from build123d import *

# Parameters (mm, degrees)
SCHIZZO1_R                   = 2.15
ESTRUSIONE_ESTRUSIONE1_DEPTH = 160


with BuildPart() as part:
    # Schizzo1 → Estrusione-Estrusione1 (new body)
    with BuildSketch(Plane(origin=(0, 0, 0), x_dir=(-1, 0, 0), z_dir=(0, 0, -1))):
        with BuildLine():
            Line((8.2, 2.5), (9, 2.5))
            ThreePointArc((9, 2.5), (9.707106781, 2.792893219), (10, 3.5))
            Line((10, 3.5), (10, 9))
            ThreePointArc((10, 9), (9.707106781, 9.707106781), (9, 10))
            Line((9, 10), (3.5, 10))
            ThreePointArc((3.5, 10), (2.792893219, 9.707106781), (2.5, 9))
            Line((2.5, 9), (2.5, 8.2))
            Line((2.5, 8.2), (4.512994231, 8.2))
            ThreePointArc((4.512994231, 8.2), (5.436873764, 7.582683432), (5.220101013, 6.492893219))
            Line((5.220101013, 6.492893219), (2.670101013, 3.942893219))
            ThreePointArc((2.670101013, 3.942893219), (2.345677664, 3.726120467), (1.962994231, 3.65))
            Line((1.962994231, 3.65), (-1.962994231, 3.65))
            ThreePointArc((-1.962994231, 3.65), (-2.345677664, 3.726120467), (-2.670101013, 3.942893219))
            Line((-2.670101013, 3.942893219), (-5.220101013, 6.492893219))
            ThreePointArc((-5.220101013, 6.492893219), (-5.436873764, 7.582683432), (-4.512994231, 8.2))
            Line((-4.512994231, 8.2), (-2.5, 8.2))
            Line((-2.5, 8.2), (-2.5, 9))
            ThreePointArc((-2.5, 9), (-2.792893219, 9.707106781), (-3.5, 10))
            Line((-3.5, 10), (-9, 10))
            ThreePointArc((-9, 10), (-9.707106781, 9.707106781), (-10, 9))
            Line((-10, 9), (-10, 3.5))
            ThreePointArc((-10, 3.5), (-9.707106781, 2.792893219), (-9, 2.5))
            Line((-9, 2.5), (-8.2, 2.5))
            Line((-8.2, 2.5), (-8.2, 4.512994231))
            ThreePointArc((-8.2, 4.512994231), (-7.582683432, 5.436873764), (-6.492893219, 5.220101013))
            Line((-6.492893219, 5.220101013), (-3.942893219, 2.670101013))
            ThreePointArc((-3.942893219, 2.670101013), (-3.726120467, 2.345677664), (-3.65, 1.962994231))
            Line((-3.65, 1.962994231), (-3.65, -1.962994231))
            ThreePointArc((-3.65, -1.962994231), (-3.726120467, -2.345677664), (-3.942893219, -2.670101013))
            Line((-3.942893219, -2.670101013), (-6.492893219, -5.220101013))
            ThreePointArc((-6.492893219, -5.220101013), (-7.582683432, -5.436873764), (-8.2, -4.512994231))
            Line((-8.2, -4.512994231), (-8.2, -2.5))
            Line((-8.2, -2.5), (-9, -2.5))
            ThreePointArc((-9, -2.5), (-9.707106781, -2.792893219), (-10, -3.5))
            Line((-10, -3.5), (-10, -9))
            ThreePointArc((-10, -9), (-9.707106781, -9.707106781), (-9, -10))
            Line((-9, -10), (-3.5, -10))
            ThreePointArc((-3.5, -10), (-2.792893219, -9.707106781), (-2.5, -9))
            Line((-2.5, -9), (-2.5, -8.2))
            Line((-2.5, -8.2), (-4.512994231, -8.2))
            ThreePointArc((-4.512994231, -8.2), (-5.436873764, -7.582683432), (-5.220101013, -6.492893219))
            Line((-5.220101013, -6.492893219), (-2.670101013, -3.942893219))
            ThreePointArc((-2.670101013, -3.942893219), (-2.345677664, -3.726120467), (-1.962994231, -3.65))
            Line((-1.962994231, -3.65), (1.962994231, -3.65))
            ThreePointArc((1.962994231, -3.65), (2.345677664, -3.726120467), (2.670101013, -3.942893219))
            Line((2.670101013, -3.942893219), (5.220101013, -6.492893219))
            ThreePointArc((5.220101013, -6.492893219), (5.436873764, -7.582683432), (4.512994231, -8.2))
            Line((4.512994231, -8.2), (2.5, -8.2))
            Line((2.5, -8.2), (2.5, -9))
            ThreePointArc((2.5, -9), (2.792893219, -9.707106781), (3.5, -10))
            Line((3.5, -10), (9, -10))
            ThreePointArc((9, -10), (9.707106781, -9.707106781), (10, -9))
            Line((10, -9), (10, -3.5))
            ThreePointArc((10, -3.5), (9.707106781, -2.792893219), (9, -2.5))
            Line((9, -2.5), (8.2, -2.5))
            Line((8.2, -2.5), (8.2, -4.512994231))
            ThreePointArc((8.2, -4.512994231), (7.582683432, -5.436873764), (6.492893219, -5.220101013))
            Line((6.492893219, -5.220101013), (3.942893219, -2.670101013))
            ThreePointArc((3.942893219, -2.670101013), (3.726120467, -2.345677664), (3.65, -1.962994231))
            Line((3.65, -1.962994231), (3.65, 1.962994231))
            ThreePointArc((3.65, 1.962994231), (3.726120467, 2.345677664), (3.942893219, 2.670101013))
            Line((3.942893219, 2.670101013), (6.492893219, 5.220101013))
            ThreePointArc((6.492893219, 5.220101013), (7.582683432, 5.436873764), (8.2, 4.512994231))
            Line((8.2, 4.512994231), (8.2, 2.5))
        make_face()
        Circle(SCHIZZO1_R, mode=Mode.SUBTRACT)
    extrude(amount=-ESTRUSIONE_ESTRUSIONE1_DEPTH)


solid = part.part
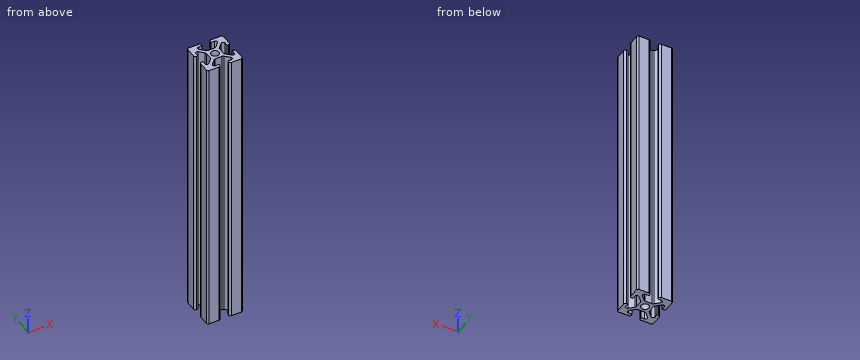
Source: CAD feature listing. Evaluate the final solid. Frame: model axes, mm. Coordinates: 2 decimals unless noted, no trailing zeros. Loops run counter-clockwise (first coordinate to the right, second up) from the corner with the lowest first, then second, coordinate; pieces in that order, holes last. Notation, with made-up numbers: (20, 83) -> (77, 83) arc R7 ccw to (77, 89) -> close; hole circle Ø8 at (-30.75, 65.25). An arc over 180 degrees is marked (long way). Answer in a Markdown table with one row per item. Add a question column.
Q1. Ray query, line 1 along Y through (x, z) = (3.75, 103.5); line 2 along X through (y, z) = (7, 128.5); line 3 along Y through (x, z) = (0, 86.5). Return the intervals inside material, ascending.
Q2. Contact query for flat-ended pins moving along their axis: pin 1 Ø1.2 at (x, z) = (0.5, 69) entering from +Y; pin 2 Ø2 at (y, z) = (0.5, 98.5) entering from -X; pin 3 Ø6 at (y, z) = (0, 44.5) entering from +X. Output: stop coordinate, or through.
Q3. Section A-A on x = 0. Return the cut outline in (y, z), and give its area (3 significant figures).
Computed values:
| question | item | result |
|---|---|---|
| 1 | line 1 | y = -10 to -8.2, -5.02 to -2.4, 2.4 to 5.02, 8.2 to 10 |
| 1 | line 2 | x = -10 to -5.49, 5.49 to 10 |
| 1 | line 3 | y = -3.65 to -2.15, 2.15 to 3.65 |
| 2 | pin 1 | stops at y = 3.65 |
| 2 | pin 2 | stops at x = -3.65 |
| 2 | pin 3 | stops at x = 9.87 |
| 3 | outline | (-3.65, 0) -> (-2.15, 0) -> (-2.15, 160) -> (-3.65, 160) -> close; (2.15, 0) -> (3.65, 0) -> (3.65, 160) -> (2.15, 160) -> close |
| 3 | area | 480 mm^2 |
